Work out the finished part from the listing and answer in its coordinate system (mm). A direction names the side the tool comes from. Give positions to 0.01 mm unless a question says otherwise; leave off trailing zeros. Loops run counter-clockwise (first coordinate to the right, second up) from the corner with the lowest first, then second, coordinate; pieces in that order, holes last. Notation, with made-up numbers: M 70,64.25 L 75,64.25 A23 cw 75,77.25 Z; hole C 82,23 d3. An arc over 180 degrees is marked long. Answer in a Markdown table with one row per item. Add a question column.
Autodesk Inventor part; units mm, degrees
ref_plane "Work Plane2" through (31.1532, -17.5901, -37) normal (0.7071, 0.7071, 0) x (-0.7071, 0.7071, 0)
ref_plane "Work Plane4" through (0.92, 19.6401, -37) normal (-1, 0, 0) x (0, 0, -1)
ref_plane "YZ Plane" through (0, 0, 0) normal (1, 0, 0) x (0, 1, 0)
sketch "Sketch1" plane through (0, 0, 0) normal (0, 0, 1) x (1, 0, 0)
  line L0 (0, 0) -> (0, 7.4776)
  line L1 (0, 7.4776) -> (-5.7, 7.4776)
  line L2 (-5.7, 7.4776) -> (-21.2563, -8.0788)
  line L3 (-21.2563, -8.0788) -> (-21.2563, -11.0788)
  line L4 (-21.2563, -11.0788) -> (-20.5492, -11.7859)
  line L5 (-20.5492, -11.7859) -> (-21.2563, -12.493)
  line L6 (-21.2563, -12.493) -> (-19.7664, -13.983)
  line L7 (-19.7664, -13.983) -> (-25.1404, -19.357)
  line L8 (-25.1404, -19.357) -> (-27.1017, -19.2987)
  line L9 (-27.1017, -19.2987) -> (-27.8088, -20.0059)
  line L10 (-27.8088, -20.0059) -> (-23.0005, -24.8142)
  line L11 (-23.0005, -24.8142) -> (-3.2015, -5.0152)
  line L12 (-1.88, 9.6426) -> (-1.2574, 11.8658)
  line L13 (-1.2574, 11.8658) -> (-2.8574, 11.8658)
  line L14 (-2.8574, 11.8658) -> (-5.5444, 9.1788)
  line L15 (-23.5149, -7.7918) -> (-6.5444, 9.1788)
  line L16 (-6.5444, 9.1788) -> (-5.5444, 9.1788)
  line L17 (-23.5149, -7.7918) -> (-23.5149, -11.7918)
  line L18 (-29.3132, -17.5901) -> (-23.5149, -11.7918)
  line L19 (-29.3132, -17.5901) -> (-30.4446, -16.4587)
  line L20 (-30.4446, -16.4587) -> (-29.4153, -15.4295)
  line L21 (-29.4153, -15.4295) -> (-30.1224, -14.7223)
  line L22 (-30.1224, -14.7223) -> (-32.668, -17.2679)
  line L23 (-32.668, -17.2679) -> (-22.9298, -27.0062)
  line L24 (-22.9298, -27.0062) -> (-1.4337, -5.5102)
  line L25 (0.92, 16.812) -> (0.92, -19.9546) construction
  line L26 (1.84, 0) -> (1.84, 7.4776)
  line L27 (1.84, 7.4776) -> (7.54, 7.4776)
  line L28 (7.54, 7.4776) -> (23.0963, -8.0788)
  line L29 (23.0963, -8.0788) -> (23.0963, -11.0788)
  line L30 (23.0963, -11.0788) -> (22.3892, -11.7859)
  line L31 (22.3892, -11.7859) -> (23.0963, -12.493)
  line L32 (23.0963, -12.493) -> (21.6064, -13.983)
  line L33 (21.6064, -13.983) -> (26.9804, -19.357)
  line L34 (26.9804, -19.357) -> (28.9417, -19.2987)
  line L35 (28.9417, -19.2987) -> (29.6488, -20.0059)
  line L36 (29.6488, -20.0059) -> (24.8405, -24.8142)
  line L37 (24.8405, -24.8142) -> (5.0415, -5.0152)
  line L38 (3.72, 9.6426) -> (3.0974, 11.8658)
  line L39 (3.0974, 11.8658) -> (4.6974, 11.8658)
  line L40 (4.6974, 11.8658) -> (7.3844, 9.1788)
  line L41 (25.3549, -7.7918) -> (8.3844, 9.1788)
  line L42 (8.3844, 9.1788) -> (7.3844, 9.1788)
  line L43 (25.3549, -7.7918) -> (25.3549, -11.7918)
  line L44 (31.1532, -17.5901) -> (25.3549, -11.7918)
  line L45 (31.1532, -17.5901) -> (32.2846, -16.4587)
  line L46 (32.2846, -16.4587) -> (31.2553, -15.4295)
  line L47 (31.2553, -15.4295) -> (31.9624, -14.7223)
  line L48 (31.9624, -14.7223) -> (34.508, -17.2679)
  line L49 (34.508, -17.2679) -> (24.7698, -27.0062)
  line L50 (24.7698, -27.0062) -> (3.2737, -5.5102)
  line L51 (-1.88, 9.6426) -> (3.72, 9.6426)
  arc A0 (3.2737, -5.5102) -> (-1.4337, -5.5102) centre (0.92, -4.1167) ccw
  arc A1 (5.0415, -5.0152) -> (1.84, 0) centre (0.92, -4.1167) ccw
  arc A2 (0, 0) -> (-3.2015, -5.0152) centre (0.92, -4.1167) ccw
  point P0 (-22.4534, -16.67)
  dimension "d1" = 5.7
  dimension "d2" = 135
  dimension "d3" = 22
  dimension "d13" = 3
  dimension "d14" = 28
  dimension "d22" = 1.6
  dimension "d23" = 3.8
  dimension "d24" = 1
  dimension "d25" = 24
  dimension "d30" = 4
  dimension "d34" = 3.6
  dimension "d36" = 1.5
  dimension "d38" = 1.6
  dimension "d47" = 1.84
  dimension "d55" = 8.2
  dimension "d56" = 1.6
  dimension "d57" = 1
  dimension "d59" = 7.6
  dimension "d61" = 1
  dimension "d62" = 6.8
  dimension "d72" = 30.4
  dimension "d74" = 13.772
  dimension "d75" = 4.2
  dimension "d76" = 5.6
  dimension "d77" = 1.8
  dimension "d78" = 1
  dimension "d80" = 90
  dimension "d81" = 7.4776
extrude "Extrusion1" add sketch "Sketch1" against normal blind 37
ref_plane "Work Plane2" through (31.1532, -17.5901, -37) normal (0.7071, 0.7071, 0) x (-0.7071, 0.7071, 0)
sketch "Sketch3" plane through (31.1532, -17.5901, -37) normal (0.7071, 0.7071, 0) x (-0.7071, 0.7071, 0)
  circle A0 centre (5.2, 18.5) radius 3
  line L0 (0, 37) -> (8.2, 37)
  line L1 (8.2, 37) -> (8.2, 0)
  point P0 (34.4667, 37)
  dimension "d65" = 18.5
  dimension "d67" = 6
extrude "Extrusion2" cut sketch "Sketch3" against normal blind 6
thread "Thread1"
ref_plane "Work Plane4" through (0.92, 19.6401, -37) normal (-1, 0, 0) x (0, 0, -1)
mirror "Mirror2" about plane through (0.92, 19.6401, -37) normal (-1, 0, 0) of "Extrusion2"
properties part number "ESCUADRA"
(1) The mould has two halves that part along Z. Classify faces 5 (the face through (-25.438, -22.376, -18.241)), 6 (the face through (-24.63, -15.84, -15.57)): pulls with the +Z half, pulls with the -Z half, needs draft (parallel to the pull), parting line crosses it, or undercut.
(2) Section C-C, the plane z = -31.5 is taken. State how many separate pieces and enclosed holes the cut face has, and give its area (3 significant figures).
(3) Each of these flat-tipped pins is pushed along its axis until it touches: P1, Ø2, axis at y = -10.5, z = -22.5, coming from the -X side; P2, Ø8, axis at y = 3, z = -14, coming from the -X side; P3, Ø4, axis at y = 7, z = -20.5, coming from the -X side. Where does it stop, or does it pass through?
(4) Which of the six approach directions +Z, -Z, +X, -X, +Y, -Y give full straight-line access (tool end or side, diameter ignored) to faces 1 (the face through (-23.515, -10, -18)), 2 (the face through (14.172, -16.409, -18.241)), 3 (the face through (-28.387, -16.664, -18.241)), 4 (the face through (15.21, -0.19, -18.24))?
(5) Consider line 1 along X through (y, z) = (-16, -28); line 2 along X through (y, z) = (-14, -33.5); line 3 along X through (y, z) = (4, -17.5). Determine where each line is inside the solid, lowest interval first. Write a range as from..to.
(6) Section A-A, the plane x = 15.5 is taken. Determine the outline of the cut face in (y, z).
(7) Section D-D, the plane x = 0.92 is taken. Determine the outline of the cut face in (y, z), and give its area (3 significant figures).
(8) Section B-B, the plane y = 1.5 is taken. Determine the outline of the cut face in (x, z).
Numbers:
| question | item | result |
|---|---|---|
| 1 | face 5 | needs draft |
| 1 | face 6 | undercut |
| 2 | separate pieces | 1 |
| 2 | enclosed holes | 2 |
| 2 | area | 392 mm² |
| 3 | P1 | stops at x = -23.51 |
| 3 | P2 | stops at x = -16.72 |
| 3 | P3 | stops at x = -10.72 |
| 4 | face 1 | +Z, -Z, -X, +Y |
| 4 | face 2 | +Z, -Z, -Y |
| 4 | face 3 | +Z, -Z, +Y |
| 4 | face 4 | +Z, -Z |
| 5 | line 1 | x = -31.4..-29.99, -27.72..-21.78, -14.19..-11.92, 13.76..16.03, 23.62..29.56, 31.83..33.24 |
| 5 | line 2 | x = -25.72..-19.78, -12.19..-9.92, 11.76..14.03, 21.62..27.56 |
| 5 | line 3 | x = -11.72..-9.18, 0..1.84, 11.02..13.56 |
| 6 | outline | M -17.74,-37 L -15.47,-37 L -15.47,0 L -17.74,0 Z; M -0.48,-37 L 2.06,-37 L 2.06,0 L -0.48,0 Z |
| 7 | outline | M -1.38,-37 L 9.64,-37 L 9.64,0 L -1.38,0 Z |
| 7 | area | 408 mm² |
| 8 | outline | M -14.22,-37 L -11.68,-37 L -11.68,0 L -14.22,0 Z; M 0,-37 L 1.84,-37 L 1.84,0 L 0,0 Z; M 13.52,-37 L 16.06,-37 L 16.06,0 L 13.52,0 Z |
